```python
from build123d import *

# Parameters (mm, degrees)
SKETCH_W        = 152
SKETCH_H        = 152
PAD_DEPTH       = 2.5
SKETCH001_R     = 8
SKETCH001_R_2   = 3.5
POCKET_DEPTH    = 5
SKETCH002_R     = 1.25
POCKET001_DEPTH = 5
CHAMFER_SIZE    = 2


with BuildPart() as part:
    # Sketch → Pad (new body)
    with BuildSketch(Plane.XY):
        Rectangle(SKETCH_W, SKETCH_H)
    extrude(amount=PAD_DEPTH)

    # Sketch001 → Pocket (cut)
    with BuildSketch(Plane.XY.offset(2.5)):
        with Locations((-55, 55)):
            Circle(SKETCH001_R)
        with Locations((-51, -60)):
            Circle(SKETCH001_R_2)
        with Locations((-55, 15)):
            Circle(SKETCH001_R)
        with Locations((0, 15)):
            Circle(SKETCH001_R)
        with Locations((0, -25)):
            Circle(SKETCH001_R)
        with Locations((0, 55)):
            Circle(SKETCH001_R)
        with Locations((-17, -60)):
            Circle(SKETCH001_R_2)
        with Locations((17, -60)):
            Circle(SKETCH001_R_2)
        with Locations((51, -60)):
            Circle(SKETCH001_R_2)
        with Locations((55, 55)):
            Circle(SKETCH001_R)
        with Locations((-55, -25)):
            Circle(SKETCH001_R)
        with Locations((55, -25)):
            Circle(SKETCH001_R)
        with Locations((55, 15)):
            Circle(SKETCH001_R)
    extrude(amount=-POCKET_DEPTH, mode=Mode.SUBTRACT)

    # Sketch002 → Pocket001 (cut)
    with BuildSketch(Plane.XY.offset(2.5)):
        with Locations((-70, 70)):
            Circle(SKETCH002_R)
        with Locations((70, 70)):
            Circle(SKETCH002_R)
        with Locations((70, -70)):
            Circle(SKETCH002_R)
        with Locations((-70, -70)):
            Circle(SKETCH002_R)
    extrude(amount=-POCKET001_DEPTH, mode=Mode.SUBTRACT)

    # Chamfer
    chamfer_edges = [part.edges().sort_by_distance(p)[0] for p in [
        (-71.25, 70, 2.5),
        (68.75, 70, 2.5),
        (68.75, -70, 2.5),
        (-71.25, -70, 2.5),
    ]]
    chamfer(chamfer_edges, length=CHAMFER_SIZE)


solid = part.part
```
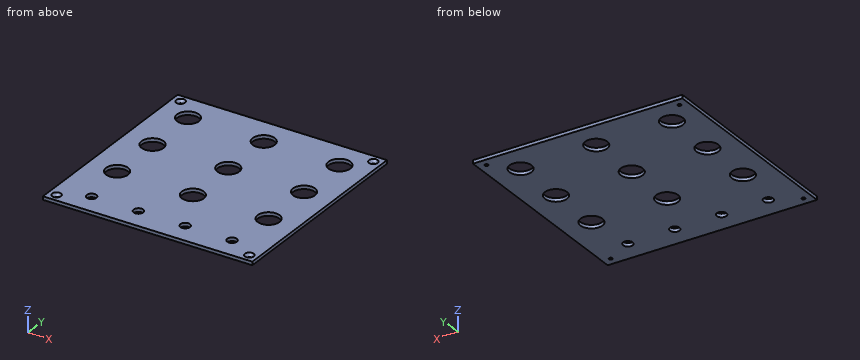
Geometry: final body of the model. Coordinates: model frame, mm. Round coordinates to 2 decimals unless told otherwise and drop trailing zeros. Loops run counter-clockwise (first coordinate to the right, second up) from the corner with the lowest first, then second, coordinate; pieces in that order, holes last. Notation, with made-up numbers: (-21.5, -23) -> (32.5, -23) arc R20 ccw to (32.5, -1) -> close; hole circle Ø7 at (78.5, 44.5). An arc over 180 degrees is marked (long way). Use one line per item in the form item = value. Start each with the question number.
1) First-contact query: P1, Ø6.5, axis at x = -51, y = -60, coming from the +Z side; P2, Ø8, axis at x = -17, y = -60, coming from the +Z side; P3, Ø4, axis at x = 70, y = -70, coming from the +Z side. Flat tips, straight axial feed; report the tip coordinate or a pass-through.
2) Section B-B on x = 17. Output: boundary loops of the cut face in (y, z), then the cut area to 4 significant figures.
3) Section A-A on z = 0.95. Give the number of separate pieces and of enclosed holes in the cut face, then the cut area to 3 significant figures.
4) Section D-D on y = -21. Output: boundary loops of the cut face in (x, z), then the cut area to 3 significant figures.
5) Line query: L1, parallel to X at y = -70, z = 0.35; L2, parallel to X at y = -69.5, z = 0.8; L3, parallel to X at y = -26, z = 0.8. Output: solid intervals per line, ascending.
6) Section C-C on y = 15. Output: boundary loops of the cut face in (x, z).
Response:
q1.P1 = through
q1.P2 = 2.5
q1.P3 = 1.25
q2.outline = (-76, 0) -> (-63.5, 0) -> (-63.5, 2.5) -> (-76, 2.5) -> close; (-56.5, 0) -> (76, 0) -> (76, 2.5) -> (-56.5, 2.5) -> close
q2.area = 362.5 mm^2
q3.separate_pieces = 1
q3.enclosed_holes = 17
q3.area = 21,100 mm^2
q4.outline = (-76, 0) -> (-61.93, 0) -> (-61.93, 2.5) -> (-76, 2.5) -> close; (-48.07, 0) -> (-6.93, 0) -> (-6.93, 2.5) -> (-48.07, 2.5) -> close; (6.93, 0) -> (48.07, 0) -> (48.07, 2.5) -> (6.93, 2.5) -> close; (61.93, 0) -> (76, 0) -> (76, 2.5) -> (61.93, 2.5) -> close
q4.area = 276 mm^2
q5.L1 = -76 to -71.25, -68.75 to 68.75, 71.25 to 76
q5.L2 = -76 to -71.47, -68.53 to 68.53, 71.47 to 76
q5.L3 = -76 to -62.94, -47.06 to -7.94, 7.94 to 47.06, 62.94 to 76
q6.outline = (-76, 0) -> (-63, 0) -> (-63, 2.5) -> (-76, 2.5) -> close; (-47, 0) -> (-8, 0) -> (-8, 2.5) -> (-47, 2.5) -> close; (8, 0) -> (47, 0) -> (47, 2.5) -> (8, 2.5) -> close; (63, 0) -> (76, 0) -> (76, 2.5) -> (63, 2.5) -> close
